Geometry check sheet. Reference: the model listing, model coordinates, mm. A direction names the side the tool comes from. Round coordinates to 2 decimals unless told otherwise and drop trailing zeros. Loops run counter-clockwise (first coordinate to the right, second up) from the corner with the lowest first, then second, coordinate; pieces in that order, holes last. Notation, with made-up numbers: (65, 7.5) -> (83, 7.5) arc R17 cw to (83, 26.5) -> close; hole circle Ø11 at (1, 55). An arc over 180 degrees is marked (long way). Use a Markdown table: item, result. Add a question column.
Q1. Material ranges on L1, parallel to Y at x = -1.5, z = -21.5; L2, parallel to Y at x = -50, z = 4.25; L3, parallel to X at y = 6, z = 10.5, recorded low to high.
Q2. Sectioned sample at D-D, the plane y = 0. Enter the section's corners in (x, z).
Q3. Set-up check for faces 1 (the face through (-1, 26, -24)), 2 (the face through (-38.118, -20.93, -0.837)): record each of +Z, -Z, +X, -X, +Y, -Y from which the full face is reachable in a straight line by a thin tool's end or side.
Q4. Sectioned sample at A-A, the plane x = -50. Enter the section's corners in (y, z), then the cut area to 3 significant figures.
Q5. Sectioned sample at C-C, the plane x = 0. Enter the section's corners in (y, z).
Q6. Release check for a two-part mould opening along X. For faces 3 (the face through (-43.323, 2.103, 6.902)), 4 (the face through (-65, -27, 7)), 5 (the face through (-1, 0, 14)) record: released by +X, released by -X, zero draft, split by the parting line, or undercut.
Q7. Gauge pin test, flat ends, axial feed: P1, Ø1, axis at x = 11.5, z = -43.5, coming from the +Y side; P2, Ø1.5, axis at x = 15, z = -9, coming from the -Y side; P3, Ø10, axis at y = -22.5, z = -7, coming from the +X side. Record the tip position at first contact, or that the pin passes through.
Q8. Sectioned sample at B-B, the plane y = -20. Enter the section's corners in (x, z).
```python
from build123d import *

# Parameters (mm, degrees)
SKETCH1_W            = 132
SKETCH1_H            = 58
SKETCH1_R            = 7
BOSS_EXTRUDE1_DEPTH  = 14
FILLET1_R            = 5
SKETCH2_R            = 8
BOSS_EXTRUDE2_DEPTH  = 10
FILLET2_R            = 5
FILLET2_OF_MIRROR1_R = 5


with BuildPart() as part:
    # Sketch1 → Boss-Extrude1 (new body)
    with BuildSketch(Plane.XY):
        Rectangle(SKETCH1_W, SKETCH1_H)
        with Locations((-50, 0)):
            Circle(SKETCH1_R, mode=Mode.SUBTRACT)
        with Locations((50, 0)):
            Circle(SKETCH1_R, mode=Mode.SUBTRACT)
    extrude(amount=BOSS_EXTRUDE1_DEPTH)

    # Fillet1
    fillet1_edges = [part.edges().sort_by_distance(p)[0] for p in [
        (66, -29, 7),
        (-66, -29, 7),
        (-66, 29, 7),
        (66, 29, 7),
    ]]
    fillet(fillet1_edges, radius=FILLET1_R)

    # Sketch2 → Boss-Extrude2 (add)
    with BuildSketch(Plane(origin=(0, -26, 0), x_dir=(-1, 0, 0), z_dir=(0, -1, 0))):
        with BuildLine():
            Line((-37.5, 0), (-18.575020612, 47.414081823))
            ThreePointArc((-18.575020612, 47.414081823), (0, 60), (18.575020612, 47.414081823))
            Line((18.575020612, 47.414081823), (37.5, 0))
            Line((37.5, 0), (-37.5, 0))
        make_face()
        with Locations(Location((0, 40, 0), (0, 0, 90))):
            Circle(SKETCH2_R, mode=Mode.SUBTRACT)
    boss_extrude2 = extrude(amount=-BOSS_EXTRUDE2_DEPTH)

    # Fillet2
    fillet2_edges = [part.edges().sort_by_distance(p)[0] for p in [
        (-37.5, -21, 0),
        (37.5, -21, 0),
    ]]
    fillet(fillet2_edges, radius=FILLET2_R)

    # Mirror1: Boss-Extrude2 across plane
    add(boss_extrude2.mirror(Plane.ZX))

    # Fillet2 of Mirror1
    fillet2_of_mirror1_edges = [part.edges().sort_by_distance(p)[0] for p in [
        (-37.5, 21, 0),
        (37.5, 21, 0),
    ]]
    fillet(fillet2_of_mirror1_edges, radius=FILLET2_OF_MIRROR1_R)


solid = part.part
```
Values:
| question | item | result |
|---|---|---|
| 1 | L1 | -26 to -16, 16 to 26 |
| 1 | L2 | -29 to -7, 7 to 29 |
| 1 | L3 | -66 to -53.61, -46.39 to 46.39, 53.61 to 66 |
| 2 | outline | (-66, 0) -> (-57, 0) -> (-57, 14) -> (-66, 14) -> close; (-43, 0) -> (43, 0) -> (43, 14) -> (-43, 14) -> close; (57, 0) -> (66, 0) -> (66, 14) -> (57, 14) -> close |
| 3 | face 1 | -Z, +X, -X, +Y |
| 3 | face 2 | -Z, -X, +Y, -Y |
| 4 | outline | (-29, 0) -> (-7, 0) -> (-7, 14) -> (-29, 14) -> close; (7, 0) -> (29, 0) -> (29, 14) -> (7, 14) -> close |
| 4 | area | 616 mm^2 |
| 5 | outline | (-29, 0) -> (-26, 0) -> (-26, -32) -> (-16, -32) -> (-16, 0) -> (16, 0) -> (16, -32) -> (26, -32) -> (26, 0) -> (29, 0) -> (29, 14) -> (-29, 14) -> close; (-26, -60) -> (-16, -60) -> (-16, -48) -> (-26, -48) -> close; (16, -60) -> (26, -60) -> (26, -48) -> (16, -48) -> close |
| 6 | face 3 | undercut |
| 6 | face 4 | released by -X |
| 6 | face 5 | zero draft |
| 7 | P1 | y = 26 |
| 7 | P2 | y = -26 |
| 7 | P3 | x = 36.89 |
| 8 | outline | (-66, 0) -> (-40.89, 0) arc R5 cw to (-36.24, -3.15) -> (-18.58, -47.41) arc R20 ccw to (18.58, -47.41) -> (36.24, -3.15) arc R5 cw to (40.89, 0) -> (66, 0) -> (66, 14) -> (-66, 14) -> close; hole circle Ø16 at (0, -40) |
